```python
from build123d import *

# Parameters (mm, degrees)
EXTRUDE_THIN1_DEPTH = 444.5
FILLET1_R           = 1.27


with BuildPart() as part:
    # Sketch1 → Extrude-Thin1 (new body)
    with BuildSketch(Plane.XY):
        with BuildLine():
            Line((0, 0), (-3.175, 0))
            ThreePointArc((-3.175, 0), (-3.594278481, 4.295332119), (-5.909507538, 7.9375))
            ThreePointArc((-5.909507538, 7.9375), (-8.224736594, 11.579667881), (-8.644015075, 15.875))
            Line((-8.644015075, 15.875), (-12.7, 15.875))
            Line((-12.7, 15.875), (-12.7, 44.45))
            Line((-12.7, 44.45), (-11.43, 44.45))
            Line((-11.43, 44.45), (-11.43, 17.145))
            Line((-11.43, 17.145), (-7.048306528, 17.145))
            ThreePointArc((-7.048306528, 17.145), (-7.232980949, 12.705393558), (-5.025332022, 8.849165321))
            ThreePointArc((-5.025332022, 8.849165321), (-2.652667269, 5.384979729), (-1.817765075, 1.27))
            Line((-1.817765075, 1.27), (0, 1.27))
            Line((0, 1.27), (0, 0))
        make_face()
    extrude(amount=-EXTRUDE_THIN1_DEPTH)

    # Fillet1
    fillet1_edges = [part.edges().sort_by_distance(p)[0] for p in [
        (-7.048306528, 17.145, -222.25),
        (-3.175, 0, -222.25),
        (-12.7, 15.875, -222.25),
    ]]
    fillet(fillet1_edges, radius=FILLET1_R)


solid = part.part
```
CAD build for the part. Positions are in the model's coordinates, mm. A direction names the side the tool comes from. Round coordinates to 2 decimals unless told otherwise and drop trailing zeros. Order: outer loops, then holes, each group sorted by start corner. A loop starts at its lowest first (then second) coordinate and runs counter-clockwise, first axis right, second up.
Q1. Slice it at A-A (y = 27). Write the cut outline in (x, z), and give its area (3 significant figures).
Q2. Which spindle directions (+Z, -Z, +X, -X, +Y, -Y) get a long thin tool onto all of the face, cutting with end or side? Do faces 1 (the flat face through (-11.43, 31, -219)), 2 (the cylindrical face through (-7.04, 12.04, -219.14)). Say none if no direction does.
Q3. Wall check: L1, parallel to X at y = 21.5, z = -169.5; L2, parallel to Y at x = -1.75, z = -194; L3, parallel to Y at x = -10, z = -283 (3 decimals). Give the ranges that are in metal, low to high.
Q4. Drop flat-ended pins along their axis: pin 1 (5 mm diameter, centred on x = -4.5, y = 9, fed in from -Z); pin 2 (1.5 mm diameter, centred on x = -11, z = -187.5, fed in from -Y) (3 decimals); pin 3 (1 mm diameter, centred on y = 32, z = -376.5, fed in from +X); pin 4 (3 mm diameter, centred on x = -4, z = -101, fed in from +Y). Give the stop position or say it passes through.
Results below:
1. outline: (-12.7, -444.5) - (-11.43, -444.5) - (-11.43, 0) - (-12.7, 0) - close
1. area: 565 mm2
2. face 1: +Z, -Z, +X, +Y
2. face 2: +Z, -Z, +X
3. L1: x = -12.7 to -11.43
3. L2: y = 0 to 1.27
3. L3: y = 15.875 to 17.145
4. pin 1: stops at z = -444.5
4. pin 2: stops at y = 15.875
4. pin 3: stops at x = -11.43
4. pin 4: stops at y = 9.35
